Build history of the part. All positions in model axes, mm. Face numbers are marked on the shaded views. A direction names the side the tool comes from. Coordinates: 2 decimals unless noted, no trailing zeros. Write each loop counter-clockwise with the first axis right and the second up, starting at its lowest first coordinate (ties: lowest second). Pieces come first, ordered by that corner, then holes.
```python
from build123d import *

# Parameters (mm, degrees)
BOSS_EXTRUDE1_DEPTH = 10
CUT_EXTRUDE1_DEPTH  = 8.5
CUT_EXTRUDE2_START  = -12
SKETCH6_R           = 1.5
CUT_EXTRUDE2_DEPTH  = 12
BOSS_EXTRUDE2_DEPTH = 2
FILLET2_R           = 0.5
FILLET3_R           = 1


with BuildPart() as part:
    # Sketch4 → Boss-Extrude1 (new body)
    with BuildSketch(Plane.XY):
        with BuildLine():
            Line((1, 0.1), (11, 0.1))
            ThreePointArc((11, 0.1), (11.707106781, 0.392893219), (12, 1.1))
            Line((12, 1.1), (12, 11.9))
            ThreePointArc((12, 11.9), (11.707106781, 12.607106781), (11, 12.9))
            Line((11, 12.9), (1, 12.9))
            ThreePointArc((1, 12.9), (0.292893219, 12.607106781), (0, 11.9))
            Line((0, 11.9), (0, 1.1))
            ThreePointArc((0, 1.1), (0.292893219, 0.392893219), (1, 0.1))
        make_face()
    extrude(amount=BOSS_EXTRUDE1_DEPTH)

    # Sketch5 → Cut-Extrude1 (cut)
    with BuildSketch(Plane.XY):
        with BuildLine():
            Line((11.445, 6.5), (10.555, 6.5))
            ThreePointArc((10.555, 6.5), (10, 5.945), (9.445, 6.5))
            Line((9.445, 6.5), (8.555, 6.5))
            ThreePointArc((8.555, 6.5), (8, 5.945), (7.445, 6.5))
            Line((7.445, 6.5), (6.555, 6.5))
            ThreePointArc((6.555, 6.5), (6, 5.945), (5.445, 6.5))
            Line((5.445, 6.5), (4.555, 6.5))
            ThreePointArc((4.555, 6.5), (4, 5.945), (3.445, 6.5))
            Line((3.445, 6.5), (2.555, 6.5))
            ThreePointArc((2.555, 6.5), (2, 5.945), (1.445, 6.5))
            Line((1.445, 6.5), (0.555, 6.5))
            ThreePointArc((0.555, 6.5), (0.392444264, 6.107555736), (0, 5.945))
            Line((0, 5.945), (0, 7.345))
            Line((0, 7.345), (12, 7.345))
            Line((12, 7.345), (12, 5.945))
            ThreePointArc((12, 5.945), (11.607555736, 6.107555736), (11.445, 6.5))
        make_face()
    extrude(amount=CUT_EXTRUDE1_DEPTH, mode=Mode.SUBTRACT)

    # Sketch6 → Cut-Extrude2 (cut)
    with BuildSketch(Plane.ZY.offset(CUT_EXTRUDE2_START)):
        with Locations((6, 3.25)):
            Circle(SKETCH6_R)
        Polygon((2, 2.65), (2, 0.1), (0, 0.1), (0, 2.15), align=None)
        Polygon((0, 12.9), (0, 10.85), (2, 10.35), (2, 12.9), align=None)
    extrude(amount=CUT_EXTRUDE2_DEPTH, mode=Mode.SUBTRACT)

    # Sketch7 → Boss-Extrude2 (add)
    with BuildSketch(Plane.ZY):
        Polygon((7.876388375, 1.1), (9.117691454, 3.25), (7.879275126, 5.395), (10, 5.395), (10, 1.1), align=None)
        Polygon((2, 1.1), (2, 5.395), (4.120724874, 5.395), (2.882308546, 3.25), (4.123611625, 1.1), align=None)
    extrude(amount=BOSS_EXTRUDE2_DEPTH)

    # Fillet2
    fillet2_edges = [part.edges().sort_by_distance(p)[0] for p in [
        (12, 2.4, 1),
        (12, 10.6, 1),
        (0, 10.6, 1),
        (0, 2.4, 1),
    ]]
    fillet(fillet2_edges, radius=FILLET2_R)

    # Fillet3
    fillet3_edges = [part.edges().sort_by_distance(p)[0] for p in [
        (6, 7.345, 0),
    ]]
    fillet(fillet3_edges, radius=FILLET3_R)


solid = part.part
```
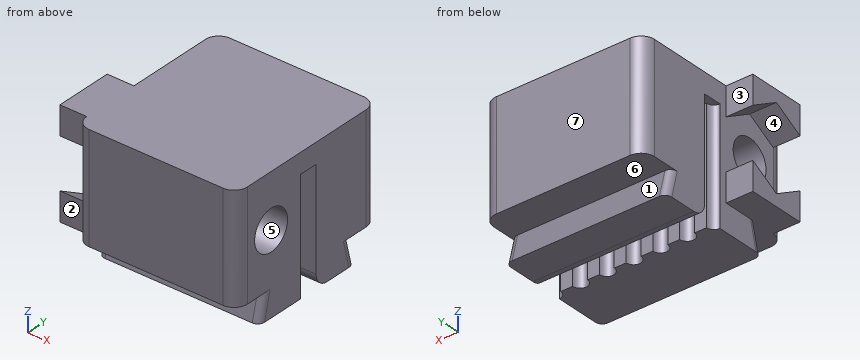
1. 3-axis set-ups, long thin cutter, end or side, ignore diameter. For the marked faces 1, 2, 3 and 4: which of +Z, -Z, +X, -X, +Y, -Y reach the whole face in a straight line?
Computed values:
face 1: +X, -X, +Y
face 2: +Z, -Z, -X, -Y
face 3: +Z, -Z, -X, +Y
face 4: -X
2. Mould opens along Y. For the marked faces 5, 6 and 7 say: +Y half, -Y half, draft (parallel to the pull), parting line (faces both ways), or undercut.
Computed values:
face 5: undercut
face 6: draft
face 7: +Y half
3. Saw through at B-B on x = 4.75. List the corners of the cut face in (y, z) (3 decimals), plus the area to 3 significant figures.
Computed values:
outline: (0.1, 2) - (2.65, 2) - (2.15, 0) - (6.5, 0) - (6.5, 8.5) - (7.345, 8.5) - (7.345, 1) arc R1 ccw to (8.345, 0) - (10.85, 0) - (10.35, 2) - (12.9, 2) - (12.9, 10) - (0.1, 10) - close; hole circle Ø3 at (3.25, 6)
area: 104 mm2
4. Saw through at A-A on z = 6. List the corners of the cut face in (x, y) (3 decimals), plus the area to 3 significant figures.
Computed values:
outline: (0, 1.1) arc R1 ccw to (1, 0.1) - (11, 0.1) arc R1 ccw to (12, 1.1) - (12, 1.75) - (0, 1.75) - close; (0, 4.75) - (12, 4.75) - (12, 5.945) arc R0.555 cw to (11.445, 6.5) - (10.555, 6.5) arc R0.555 cw to (9.445, 6.5) - (8.555, 6.5) arc R0.555 cw to (7.445, 6.5) - (6.555, 6.5) arc R0.555 cw to (5.445, 6.5) - (4.555, 6.5) arc R0.555 cw to (3.445, 6.5) - (2.555, 6.5) arc R0.555 cw to (1.445, 6.5) - (0.555, 6.5) arc R0.555 cw to (0, 5.945) - close; (0, 7.345) - (12, 7.345) - (12, 11.9) arc R1 ccw to (11, 12.9) - (1, 12.9) arc R1 ccw to (0, 11.9) - close
area: 104 mm2
5. Saw through at C-C on y = 4.5. List the corners of the cut face in (x, z).
Computed values:
outline: (-2, 2) - (0, 2) - (0, 0) - (12, 0) - (12, 5.17) - (0, 5.17) - (0, 3.6) - (-2, 3.6) - close; (-2, 8.4) - (0, 8.4) - (0, 6.83) - (12, 6.83) - (12, 10) - (-2, 10) - close
6. Flat gauge pins, fed straight in: pin 1 (0.7 mm diameter, centred on x = 7.5, y = 6.5, fed in from -Z); pin 2 (0.9 mm diameter, centred on x = 4, y = 11.5, fed in from -Z); pin 3 (5 mm diameter, centred on y = 8, z = 5, fed in from -X); pin 4 (2 mm diameter, centred on x = -0.5, z = 3.5, fed in from +Y). Where does each tip first touch, or does it go through?
Computed values:
pin 1: stops at z = 0
pin 2: stops at z = 2
pin 3: stops at x = 0
pin 4: stops at y = 12.77
7. Probe line 1 along Y through (x, z) = (4, 6) (3 decimals); line 2 along Y through (x, z) = (9.25, 6) (3 decimals); line 3 along Y through (x, z) = (5.25, 4) (3 decimals). List the from-to ranges inside material, lowest first.
Computed values:
line 1: y = 0.1 to 1.75, 4.75 to 5.945, 7.345 to 12.9
line 2: y = 0.1 to 1.75, 4.75 to 6.5, 7.345 to 12.9
line 3: y = 0.1 to 6.5, 7.345 to 12.9
